from build123d import *

# Parameters (mm, degrees)
SKETCH1_R           = 18.5
BOSS_EXTRUDE1_DEPTH = 24
SKETCH2_R           = 17.25
BOSS_EXTRUDE2_DEPTH = 45
SKETCH3_R           = 6
BOSS_EXTRUDE3_DEPTH = 6
SKETCH4_R           = 3
BOSS_EXTRUDE4_DEPTH = 15
CUT_EXTRUDE1_START  = -12
CUT_EXTRUDE1_DEPTH  = 12
SKETCH6_R           = 1.5
CUT_EXTRUDE2_DEPTH  = 3


with BuildPart() as part:
    # Sketch1 → Boss-Extrude1 (new body)
    with BuildSketch(Plane.XY):
        Circle(SKETCH1_R)
    extrude(amount=BOSS_EXTRUDE1_DEPTH)

    # Sketch2 → Boss-Extrude2 (add)
    with BuildSketch(Plane(origin=(0, 0, 0), x_dir=(-1, 0, 0), z_dir=(0, 0, -1))):
        with Locations(Location((0, 0, 0), (0, 0, 180))):
            Circle(SKETCH2_R)
    extrude(amount=BOSS_EXTRUDE2_DEPTH)

    # Sketch3 → Boss-Extrude3 (add)
    with BuildSketch(Plane.XY.offset(24)):
        with Locations((0, 7)):
            Circle(SKETCH3_R)
    extrude(amount=BOSS_EXTRUDE3_DEPTH)

    # Sketch4 → Boss-Extrude4 (add)
    with BuildSketch(Plane.XY.offset(30)):
        with Locations((0, 7)):
            Circle(SKETCH4_R)
    extrude(amount=BOSS_EXTRUDE4_DEPTH)

    # Sketch5 → Cut-Extrude1 (cut)
    with BuildSketch(Plane.XY.offset(45).offset(CUT_EXTRUDE1_START)):
        with BuildLine():
            ThreePointArc((1.658312395, 9.5), (0, 10), (-1.658312395, 9.5))
            Line((-1.658312395, 9.5), (0, 9.5))
            Line((0, 9.5), (1.658312395, 9.5))
        make_face()
    extrude(amount=CUT_EXTRUDE1_DEPTH, mode=Mode.SUBTRACT)

    # Sketch6 → Cut-Extrude2 (cut)
    with BuildSketch(Plane.XY.offset(24)):
        with Locations((7.75, 13.423393759)):
            Circle(SKETCH6_R)
        with Locations((15.5, 0)):
            Circle(SKETCH6_R)
        with Locations((7.75, -13.423393759)):
            Circle(SKETCH6_R)
        with Locations((-7.75, -13.423393759)):
            Circle(SKETCH6_R)
        with Locations((-15.5, 0)):
            Circle(SKETCH6_R)
        with Locations((-7.75, 13.423393759)):
            Circle(SKETCH6_R)
    extrude(amount=-CUT_EXTRUDE2_DEPTH, mode=Mode.SUBTRACT)


solid = part.part
Part model, mm, in its own coordinate system. A direction names the side the tool comes from. Coordinates: 2 decimals unless noted, no trailing zeros. Loops run counter-clockwise (first coordinate to the right, second up) from the corner with the lowest first, then second, coordinate; pieces in that order, holes last. Notation, with made-up numbers: (25.5, 26) -> (83.5, 26) arc R23 ccw to (83.5, 61) -> close; hole circle Ø3 at (-15.5, 69). An arc over 180 degrees is marked (long way). Use a Markdown table: item, result. Add a question column.
Item 1: Probe probe 1 along Y at (x, z) = (7.75, 22.2); probe 2 along Z at (x, y) = (-11, 8); probe 3 along Y at (x, z) = (-14, -7). List the from-to ranges inside material, lowest first.
Item 2: Flat gauge pins, fed straight in: P1, Ø5, axis at x = 2, z = -20.5, coming from the -Y side; P2, Ø3, axis at y = -13, z = 12.5, coming from the +X side; P3, Ø10, axis at x = 7, z = 14, coming from the -Y side. Where does each tip first touch, or does it go through?
Item 3: Pull direction X, two halves, no side cores. Call faces 4 (the cylindrical face through (7.42, 11.96, 22.52)), 5 (the flat face through (0, 0, -45)), 6 (the cylindrical face through (-0.65, 4.07, 37.39)): +X half, -X half, draft (parallel to the pull), parting line (faces both ways), or undercut.
Item 4: Band-saw the part on B-B on x = -15.5. Write the cut outline in (y, z), plus the area to 3 significant figures.
Item 5: Band-saw the part on C-C on z = -21.5. Write the cut outline in (x, y).
Item 6: Band-saw the part on A-A on y = 0. Write the cut outline in (x, z), plus the area to 3 significant figures.
Item 7: Which spindle directions (+Z, -Z, +X, -X, +Y, -Y) get a long thin tool onto all of the face, cutting with end or side? Do faces 1 (the cylindrical face through (-17.233, -0.758, -22.185)), 2 (the cylindrical face through (6.644, -12.41, 22.521)), 3 (the flat face through (0, 9.5, 39)). Say none if no direction does.
Item 8: Band-saw the part on D-D on x = 7.75. Write the cut outline in (y, z).
Geometry says:
| question | item | result |
|---|---|---|
| 1 | probe 1 | -16.8 to -14.92, -11.92 to 11.92, 14.92 to 16.8 |
| 1 | probe 2 | -45 to 24 |
| 1 | probe 3 | -10.08 to 10.08 |
| 2 | P1 | y = -17.25 |
| 2 | P2 | x = 14.49 |
| 2 | P3 | y = -18.39 |
| 3 | face 4 | undercut |
| 3 | face 5 | draft |
| 3 | face 6 | parting line |
| 4 | outline | (-10.1, 0) -> (-7.57, 0) -> (-7.57, -45) -> (7.57, -45) -> (7.57, 0) -> (10.1, 0) -> (10.1, 24) -> (1.5, 24) -> (1.5, 21) -> (-1.5, 21) -> (-1.5, 24) -> (-10.1, 24) -> close |
| 4 | area | 1,160 mm² |
| 5 | outline | circle Ø34.5 at (0, 0) |
| 6 | outline | (-18.5, 0) -> (-17.25, 0) -> (-17.25, -45) -> (17.25, -45) -> (17.25, 0) -> (18.5, 0) -> (18.5, 24) -> (17, 24) -> (17, 21) -> (14, 21) -> (14, 24) -> (-14, 24) -> (-14, 21) -> (-17, 21) -> (-17, 24) -> (-18.5, 24) -> close |
| 6 | area | 2,420 mm² |
| 7 | face 1 | -Z |
| 7 | face 2 | +Z |
| 7 | face 3 | +Z, +X, -X, +Y |
| 8 | outline | (-16.8, 0) -> (-15.41, 0) -> (-15.41, -45) -> (15.41, -45) -> (15.41, 0) -> (16.8, 0) -> (16.8, 24) -> (14.92, 24) -> (14.92, 21) -> (11.92, 21) -> (11.92, 24) -> (-11.92, 24) -> (-11.92, 21) -> (-14.92, 21) -> (-14.92, 24) -> (-16.8, 24) -> close |
